For this review, take the finished solid that the model builds, in its own axes (mm). Give positions to 0.01 mm unless a question says otherwise; leave off trailing zeros. Loops run counter-clockwise (first coordinate to the right, second up) from the corner with the lowest first, then second, coordinate; pieces in that order, holes last. Notation, with made-up numbers: (18.25, 57.5) - (27.25, 57.5) arc R7 ccw to (27.25, 61.5) - close; hole circle Ø9 at (51, 59). An arc over 180 degrees is marked (long way). Use CSV: the item, a comma, the result in double quotes. Start each with the question number.
1. Take a section at A-A on y = -7. Give the boundary of the cut face in (x, z) (3 decimals), plus the area to 3 significant figures.
2. Wall thickness on line 1 (Y direction, x = -3, z = 0.35); line 2 (Y direction, x = 190.5, z = 1.5); line 3 (Y direction, x = 16, z = 2.15): over which ranges is each line inside the solid? List them lowest first.
3. For pin 1 (1 mm diameter, centred on x = 125.5, y = -15, fed in from -Z); pin 2 (1.6 mm diameter, centred on x = -4, z = 1.5, fed in from +Y); pin 3 (1.6 mm diameter, centred on y = -40, z = 1.5, fed in from -X); pin 4 (1 mm diameter, centred on y = -80.5, z = 1.5, fed in from +X), all flat-tipped, find the tip position at first contact; note any pin that passes through.
```python
from build123d import *

# Parameters (mm, degrees)
BOSS_EXTRUDE1_DEPTH = 3.175


with BuildPart() as part:
    # Sketch1 → Boss-Extrude1 (new body)
    with BuildSketch(Plane.XY):
        with BuildLine():
            Line((0, 0), (0, -12.7))
            Line((0, -12.7), (-12.7, -12.7))
            Line((-12.7, -12.7), (-12.7, -31.75))
            Line((-12.7, -31.75), (-6.35, -31.75))
            Line((-6.35, -31.75), (-6.35, -19.05))
            Line((-6.35, -19.05), (0, -19.05))
            Line((0, -19.05), (0, -69.85))
            Line((0, -69.85), (-12.7, -69.85))
            Line((-12.7, -69.85), (-12.7, -88.9))
            Line((-12.7, -88.9), (-6.35, -88.9))
            Line((-6.35, -88.9), (-6.35, -76.2))
            Line((-6.35, -76.2), (0, -76.2))
            Line((0, -76.2), (0, -107.95))
            add(Edge.make_bspline(
                [(0, -107.95), (64.972882445, -118.248903815), (107.260828457, -42.040801067), (176.720157179, -14.882540639), (202.4483901, -17.949390151)],
                knots=[0, 0, 0, 0, 0.687412436, 0.974132151, 0.974132151, 0.974132151, 0.974132151], degree=3))
            ThreePointArc((202.4483901, -17.949390151), (207.416027581, -16.392461261), (209.55, -11.644028737))
            Line((209.55, -11.644028737), (209.55, 6.35))
            Line((209.55, 6.35), (203.2, 6.35))
            Line((203.2, 6.35), (203.2, 0))
            Line((203.2, 0), (0, 0))
        make_face()
    extrude(amount=BOSS_EXTRUDE1_DEPTH)


solid = part.part
```
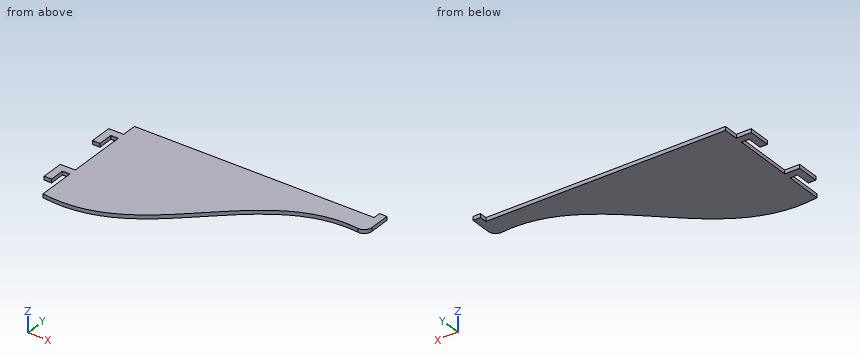
Check result:
1,outline,"(0, 0) - (209.55, 0) - (209.55, 3.175) - (0, 3.175) - close"
1,area,"665 mm²"
2,line 1,"y = -76.2 to -69.85, -19.05 to -12.7"
2,line 2,"y = -17.3 to 0"
2,line 3,"y = -109.24 to 0"
3,pin 1,"stops at z = 0"
3,pin 2,"stops at y = -12.7"
3,pin 3,"stops at x = 0"
3,pin 4,"stops at x = 85.27"
